Source: CAD feature listing. Evaluate the final solid. Frame: model axes, mm. A direction names the side the tool comes from. Round coordinates to 2 decimals unless told otherwise and drop trailing zeros. Write each loop counter-clockwise with the first axis right and the second up, starting at its lowest first coordinate (ties: lowest second). Pieces come first, ordered by that corner, then holes. Notation, with made-up numbers: M 29.5,66 L 52.5,66 A24 ccw 52.5,79 Z; hole C -4.75,34 d1. An arc over 180 degrees is marked long. Answer in a Markdown table with one row per item. Add a question column.
Item 1: Mould query, pull axis X, two halves, no side actions, for faces 1 (the face through (-79.375, -197, 82)), 2 (the face through (-95, -22.225, 82)), 3 (the face through (41.275, -6, 82)). Classes: released by +X, released by -X, zero draft, split by the parting line, or undercut.
Item 2: Set-up query: faces 4 (the face through (77.3, -196.9, 16)), 5 (the face through (-91, -94, -101.6)), 6 (the face through (-20.107, -197, -64)), 7 (the face through (41.275, -197, 82)), 8 (the face through (-95, -142.875, 82)). Return all of +Z, -Z, +X, -X, +Y, -Y with unobstructed straight access to the full face (end or side cutting, diameter ignored); none if empty.
Item 3: Cut plane A-A on x = -8.5. Return loops of the section in (y, z), and give its area (3 significant figures).
Item 4: Cut plane B-B on y = -28. Return loops of the section in (x, z).
Item 5: Cut plane C-C on z = -49. Return loops of the section in (x, y).
Item 6: Cut plane D-D on x = -59.5. Return loops of the section in (y, z).
Item 7: Contact query for flat-ended pins moving along their axis: pin 1 (10 mm diameter, centred on x = 74, z = 71, fed in from -Y); pin 2 (14 mm diameter, centred on x = -57.5, y = -3.5, fed in from +Z). Output: stop coordinate, or through.
Item 8: Material intervals for probe 1 along X at (y, z) = (-191.5, 74.5) (3 decimals); probe 2 along X at (y, z) = (-182, 24.5); probe 3 along Y at (x, z) = (51, -56.5), sorted ascending.
from build123d import *

# Parameters (mm, degrees)
F0_W      = 203.2
F0_H      = 203.2
F1_DEPTH  = 203.2
F2_W      = 177.8
F2_H      = 177.8
F3_DEPTH  = 203.2
F4_W      = 50.8
F4_H      = 76.2
F5_DEPTH  = 25.4
F6_W      = 38.1
F6_H      = 38.1
F7_DEPTH  = 25.4
F8_W      = 38.1
F8_H      = 38.1
F9_DEPTH  = 25.4
F10_W     = 38.1
F10_H     = 38.1
F11_DEPTH = 25.4
F12_W     = 38.1
F12_H     = 38.1
F13_DEPTH = 25.4
F14_R     = 19.05
F15_DEPTH = 25.4


with BuildPart() as f1:
    # F0 (on Front) → F1 (new body)
    with BuildSketch(Plane.XZ):
        Rectangle(F0_W, F0_H)
    extrude(amount=F1_DEPTH)

    # F2 (on face) → F3 (cut)
    with BuildSketch(Plane.XY.offset(101.6)):
        with Locations((0, -101.6)):
            Rectangle(F2_W, F2_H)
    extrude(amount=-F3_DEPTH, mode=Mode.SUBTRACT)

    # F4 (on face) → F5 (cut)
    with BuildSketch(Plane.XZ.offset(203.2)):
        with Locations((5.292703, -63.5)):
            Rectangle(F4_W, F4_H)
    extrude(amount=-F5_DEPTH, mode=Mode.SUBTRACT)

    # F6 (on face) → F7 (cut)
    with BuildSketch(Plane.XZ.offset(203.2)):
        with Locations((-60.325, 82.55)):
            Rectangle(F6_W, F6_H)
        with Locations((0, 82.55)):
            Rectangle(F6_W, F6_H)
        with Locations((60.325, 82.55)):
            Rectangle(F6_W, F6_H)
    extrude(amount=-F7_DEPTH, mode=Mode.SUBTRACT)

    # F8 (on face) → F9 (cut)
    with BuildSketch(Plane.YZ.offset(101.6)):
        with Locations((-161.925, 82.55)):
            Rectangle(F8_W, F8_H)
        with Locations((-101.6, 82.55)):
            Rectangle(F8_W, F8_H)
        with Locations((-41.275, 82.55)):
            Rectangle(F8_W, F8_H)
    extrude(amount=-F9_DEPTH, mode=Mode.SUBTRACT)

    # F10 (on face) → F11 (cut)
    with BuildSketch(Plane(origin=(0, 0, 0), x_dir=(-1, 0, 0), z_dir=(0, 1, 0))):
        with Locations((-60.325, 82.55)):
            Rectangle(F10_W, F10_H)
        with Locations((0, 82.55)):
            Rectangle(F10_W, F10_H)
        with Locations((60.325, 82.55)):
            Rectangle(F10_W, F10_H)
    extrude(amount=-F11_DEPTH, mode=Mode.SUBTRACT)

    # F12 (on face) → F13 (cut)
    with BuildSketch(Plane(origin=(-101.6, 0, 0), x_dir=(0, -1, 0), z_dir=(-1, 0, 0))):
        with Locations((41.275, 82.55)):
            Rectangle(F12_W, F12_H)
        with Locations((101.6, 82.55)):
            Rectangle(F12_W, F12_H)
        with Locations((161.925, 82.55)):
            Rectangle(F12_W, F12_H)
    extrude(amount=-F13_DEPTH, mode=Mode.SUBTRACT)

    # F14 (on face) → F15 (cut)
    with BuildSketch(Plane.XZ.offset(203.2)):
        with Locations((-64.062351, 24.935062)):
            Circle(F14_R)
        with Locations((59.688135, 23.263682)):
            Circle(F14_R)
    extrude(amount=-F15_DEPTH, mode=Mode.SUBTRACT)


solid = f1.part
Results below:
| question | item | result |
|---|---|---|
| 1 | face 1 | undercut |
| 1 | face 2 | zero draft |
| 1 | face 3 | undercut |
| 2 | face 4 | -Y |
| 2 | face 5 | -Z, +X, -X, +Y, -Y |
| 2 | face 6 | -Z, -Y |
| 2 | face 7 | +Z, +Y, -Y |
| 2 | face 8 | +Z, +X, -X |
| 3 | outline | M -203.2,-25.4 L -190.5,-25.4 L -190.5,63.5 L -203.2,63.5 Z; M -12.7,-101.6 L 0,-101.6 L 0,63.5 L -12.7,63.5 Z |
| 3 | area | 3,230 mm2 |
| 4 | outline | M -101.6,-101.6 L -88.9,-101.6 L -88.9,63.5 L -101.6,63.5 Z; M 88.9,-101.6 L 101.6,-101.6 L 101.6,63.5 L 88.9,63.5 Z |
| 5 | outline | M -101.6,-203.2 L -20.11,-203.2 L -20.11,-190.5 L -88.9,-190.5 L -88.9,-12.7 L 88.9,-12.7 L 88.9,-190.5 L 30.69,-190.5 L 30.69,-203.2 L 101.6,-203.2 L 101.6,0 L -101.6,0 Z |
| 6 | outline | M -203.2,-101.6 L -190.5,-101.6 L -190.5,6.44 L -203.2,6.44 Z; M -203.2,43.43 L -190.5,43.43 L -190.5,63.5 L -203.2,63.5 Z; M -12.7,-101.6 L 0,-101.6 L 0,63.5 L -12.7,63.5 Z |
| 7 | pin 1 | through |
| 7 | pin 2 | z = 63.5 |
| 8 | probe 1 | -101.6 to -79.375, -41.275 to -19.05, 19.05 to 41.275, 79.375 to 101.6 |
| 8 | probe 2 | -101.6 to -88.9, 88.9 to 101.6 |
| 8 | probe 3 | -203.2 to -190.5, -12.7 to 0 |
